```python
from build123d import *

# Parameters (mm, degrees)
SKETCH_1_R      = 1.5
EXTRUDE_1_DEPTH = 4
SKETCH_3_R      = 1.5
SKETCH_3_W      = 42
SKETCH_3_H      = 29
EXTRUDE_2_DEPTH = 5
FILLET_1_R      = 3
FILLET_2_R      = 3


with BuildPart() as part:
    # 草图1 → 凸台-拉伸1 (new body)
    # profile 1 of 3: a face of its own
    with BuildSketch(Plane(origin=(0, 0, 0), x_dir=(1, 0, 0), z_dir=(0, 1, 0))):
        Polygon((0, 0), (31.2, 0), (31.2, -34), (38.7, -34), (38.7, 5), (0, 5), align=None)
        with Locations(Location((34.95, -29, 0), (0, 0, 270))):
            Circle(SKETCH_1_R, mode=Mode.SUBTRACT)
    # profile 2 of 3: a face of its own
    with BuildSketch(Plane(origin=(0, 0, 0), x_dir=(1, 0, 0), z_dir=(0, 1, 0))):
        with BuildLine():
            Line((-31.2, 0), (0, 0))
            Line((0, 0), (0, 5))
            Line((0, 5), (-34.95, 5))
            Line((-34.95, 5), (-34.95, -27.5))
            ThreePointArc((-34.95, -27.5), (-33.889339828, -27.939339828), (-33.45, -29))
            ThreePointArc((-33.45, -29), (-33.889339828, -30.060660172), (-34.95, -30.5))
            Line((-34.95, -30.5), (-34.95, -34))
            Line((-34.95, -34), (-31.2, -34))
            Line((-31.2, -34), (-31.2, 0))
        make_face()
    # profile 3 of 3: a face of its own
    with BuildSketch(Plane(origin=(0, 0, 0), x_dir=(1, 0, 0), z_dir=(0, 1, 0))):
        with BuildLine():
            Line((-34.95, -27.5), (-34.95, 5))
            Line((-34.95, 5), (-38.7, 5))
            Line((-38.7, 5), (-38.7, -34))
            Line((-38.7, -34), (-34.95, -34))
            Line((-34.95, -34), (-34.95, -30.5))
            ThreePointArc((-34.95, -30.5), (-36.45, -29), (-34.95, -27.5))
        make_face()
    extrude(amount=EXTRUDE_1_DEPTH)

    # 草图3 → 凸台-拉伸2 (add)
    with BuildSketch(Plane(origin=(0, 0, -5), x_dir=(-1, 0, 0), z_dir=(0, 0, -1))):
        Polygon((-27, 2), (-27, -12.5), (-27, -15.5), (27, -15.5), (27, -12.5), (27, 2), (27, 16.5), (27, 19.5), (-27, 19.5), (-27, 16.5), align=None)
        with Locations((-24, 13.3)):
            Circle(SKETCH_3_R, mode=Mode.SUBTRACT)
        with Locations((24, 13.3)):
            Circle(SKETCH_3_R, mode=Mode.SUBTRACT)
        with Locations((24, -9.3)):
            Circle(SKETCH_3_R, mode=Mode.SUBTRACT)
        with Locations((-24, -9.3)):
            Circle(SKETCH_3_R, mode=Mode.SUBTRACT)
        with Locations((0, 2)):
            Rectangle(SKETCH_3_W, SKETCH_3_H, mode=Mode.SUBTRACT)
    extrude(amount=EXTRUDE_2_DEPTH)

    # 圆角1
    fillet_1_edges = [part.edges().sort_by_distance(p)[0] for p in [
        (27, -15.5, -7.5),
        (27, 19.5, -7.5),
        (-27, -15.5, -7.5),
        (-38.7, 2, -5),
        (-27, 19.5, -7.5),
        (-27, 2, -5),
        (38.7, 2, -5),
        (27, 2, -5),
    ]]
    fillet(fillet_1_edges, radius=FILLET_1_R)

    # 圆角2
    fillet_2_edges = [part.edges().sort_by_distance(p)[0] for p in [
        (38.7, 2, 34),
        (31.2, 2, 34),
        (-31.2, 2, 34),
        (-38.7, 2, 34),
    ]]
    fillet(fillet_2_edges, radius=FILLET_2_R)


solid = part.part
```
Model file for the job. Use its own axes, mm. A direction names the side the tool comes from. Give positions to 0.01 mm unless a question says otherwise; leave off trailing zeros. Loops run counter-clockwise (first coordinate to the right, second up) from the corner with the lowest first, then second, coordinate; pieces in that order, holes last. Notation, with made-up numbers: (-19.5, -38.5) - (17.5, -38.5) arc R18 cw to (17.5, -27.5) - close; hole circle Ø1 at (36, 9.5). An arc over 180 degrees is marked (long way). One line per item, written item: value. Start each with the question number.
1. Slice it at C-C (x = 19). List the corners of the cut face in (y, z).
2. Pin check, flat tips, straight feed: pin 1 (8 mm diameter, centred on x = 3.5, y = 10.5, fed in from +Z); pin 2 (1.2 mm diameter, centred on x = -5.5, y = 1.5, fed in from +Z); pin 3 (2.5 mm diameter, centred on y = 7, z = -8, fed in from +X); pin 4 (5.5 mm diameter, centred on y = 4, z = -7.5, fed in from -X). Stop position of each tip, or through.
3. Which spindle directions (+Z, -Z, +X, -X, +Y, -Y) get a long thin tool onto all of the face, cutting with end or side? Do faces 1 (the flat face through (0, 2, 0)), 2 (the flat face through (0, 18, -5)), 3 (the flat face through (0, 2, -5)). Say none if no direction does.
4. Slice it at B-B (z = 8). List the corners of the cut face in (x, y).
5. Probe L1, parallel to Y at x = -24, z = -8; L2, parallel to X at y = 0.8, z = 29; L3, parallel to X at y = -6, z = -6.5. List the from-to ranges inside material, lowest first. Write a range as from..to.
6. Slice it at A-A (y = -1). List the corners of the cut face in (x, z).
7. Slice it at D-D (y = -9.3). List the corners of the cut face in (x, z).
8. Pull direction X, two halves, no side cores. Call faces 4 (the cylindrical face through (37.8, 2.03, -4.14)), 5 (the cylindrical face through (24.325, -10.764, -7.465)), 6 (the flat face through (-31.2, 2, 16)), 7 (the flat face through (33, 2, -5)): pulls with the +X half, pulls with the -X half, needs draft (parallel to the pull), parting line crosses it, or undercut.
Solution:
1. outline: (-15.5, -10) - (-12.5, -10) - (-12.5, -5) - (-15.5, -5) - close; (0, -5) - (4, -5) - (4, 0) - (0, 0) - close; (16.5, -10) - (19.5, -10) - (19.5, -5) - (16.5, -5) - close
2. pin 1: passes through
2. pin 2: stops at z = 0
2. pin 3: stops at x = 27
2. pin 4: stops at x = -36.9
3. face 1: +Z, +Y, -Y
3. face 2: +Z, +X, -X, +Y
3. face 3: -Z
4. outline: (-38.7, 0) - (-31.2, 0) - (-31.2, 4) - (-38.7, 4) - close; (31.2, 0) - (38.7, 0) - (38.7, 4) - (31.2, 4) - close
5. L1: y = -15.5..-10.8, -7.8..11.8, 14.8..19.5
5. L2: x = -38.7..-36.45, -33.45..-31.2, 31.2..33.45, 36.45..38.7
5. L3: x = -27..-21, 21..27
6. outline: (-27, -10) - (-21, -10) - (-21, -5) - (-27, -5) - close; (21, -10) - (27, -10) - (27, -5) - (21, -5) - close
7. outline: (-27, -10) - (-25.5, -10) - (-25.5, -5) - (-27, -5) - close; (-22.5, -10) - (-21, -10) - (-21, -5) - (-22.5, -5) - close; (21, -10) - (22.5, -10) - (22.5, -5) - (21, -5) - close; (25.5, -10) - (27, -10) - (27, -5) - (25.5, -5) - close
8. face 4: pulls with the +X half
8. face 5: undercut
8. face 6: undercut
8. face 7: needs draft
